```python
from build123d import *

# Parameters (mm, degrees)
SKETCH7_W                       = 41.275
SKETCH7_H                       = 28.575
BOSS_EXTRUDE2_DEPTH             = 50.8
SKETCH31_R                      = 9.525
CUT_EXTRUDE1_DEPTH              = 6.35
FILLET3_R                       = 0.127
F_8_32_TAPPED_HOLE1_D           = 3.4544
F_8_32_TAPPED_HOLE1_DEPTH       = 10.16
F_8_32_TAPPED_HOLE1_TIP         = 1.037806461
F_17_0_173_DIAMETER_HOLE1_D     = 4.3942
F_46_0_081_DIAMETER_HOLE1_D     = 2.0574
F_46_0_081_DIAMETER_HOLE1_DEPTH = 19.066894681
F_46_0_081_DIAMETER_HOLE1_TIP   = 0.618105319


with BuildPart() as part:
    # Sketch7 → Boss-Extrude2 (new body)
    with BuildSketch(Plane(origin=(0, 0, 0), x_dir=(1, 0, 0), z_dir=(0, 1, 0))):
        with Locations((-1.5875, -7.9375)):
            Rectangle(SKETCH7_W, SKETCH7_H)
    extrude(amount=BOSS_EXTRUDE2_DEPTH)

    # Sketch31 → Cut-Extrude1 (cut)
    with BuildSketch(Plane(origin=(0, 0, -6.35), x_dir=(-1, 0, 0), z_dir=(0, 0, -1))):
        with Locations((1.5875, 25.4)):
            Circle(SKETCH31_R)
    extrude(amount=-CUT_EXTRUDE1_DEPTH, mode=Mode.SUBTRACT)

    # Sketch24 → Port Manifold (revolve, cut)
    with BuildSketch(Plane.ZY.offset(1.5875)):
        with BuildLine():
            Line((22.225, 25.4), (22.225, 33.1978))
            Line((22.225, 33.1978), (15.0368, 33.1978))
            Line((15.0368, 33.1978), (14.04146205, 32.9311))
            Line((14.04146205, 32.9311), (8.2804, 32.9311))
            ThreePointArc((8.2804, 32.9311), (8.136715902, 32.871584098), (8.0772, 32.7279))
            Line((8.0772, 32.7279), (8.0772, 29.2735))
            Line((8.0772, 29.2735), (7.637259095, 29.0195))
            Line((7.637259095, 29.0195), (4.7752, 29.0195))
            ThreePointArc((4.7752, 29.0195), (4.631515902, 28.959984098), (4.572, 28.8163))
            Line((4.572, 28.8163), (4.572, 26.034032808))
            Line((4.572, 26.034032808), (3.111576387, 26.04897))
            Line((3.111576387, 26.04897), (-0.714966433, 28.258225527))
            Line((-0.714966433, 28.258225527), (-0.714966433, 25.4))
            Line((-0.714966433, 25.4), (22.225, 25.4))
        make_face()
    revolve(axis=Axis((-1.5875, 25.4, -0.714966433), (0, 0, 1)), mode=Mode.SUBTRACT)

    # Fillet3
    fillet3_edges = [part.edges().sort_by_distance(p)[0] for p in [
        (-1.5875, 24.765967192, 4.572),
    ]]
    fillet(fillet3_edges, radius=FILLET3_R)

    # #8-32 Tapped Hole1
    with Locations(Plane.XY.offset(22.225)):
        with Locations((9.7155, 25.4)):
            Hole(F_8_32_TAPPED_HOLE1_D / 2, depth=F_8_32_TAPPED_HOLE1_DEPTH)
            with Locations((0, 0, -(F_8_32_TAPPED_HOLE1_DEPTH + F_8_32_TAPPED_HOLE1_TIP / 2))):  # 118° drill point
                Cone(0, F_8_32_TAPPED_HOLE1_D / 2, F_8_32_TAPPED_HOLE1_TIP, mode=Mode.SUBTRACT)

    # Sketch29 → 1/8 NPT Tapped Hole1 (revolve, cut)
    with BuildSketch(Plane(origin=(-1.5875, 0, 7.9375), x_dir=(0, 0, -1), z_dir=(1, 0, 0))):
        Polygon((0, 0), (0, 14.217468714), (4.2164, 11.684), (4.2164, 6.858), (4.537401096, 6.858), (4.7427388, 0), align=None)
    revolve(axis=Axis((-1.5875, -6.35, 7.9375), (0, 1, 0)), mode=Mode.SUBTRACT)

    # #17 (0.173) Diameter Hole1 (through all)
    with Locations(Plane.ZY.offset(22.225)):
        with Locations((6.35, 44.45), (15.875, 44.45)):
            Hole(F_17_0_173_DIAMETER_HOLE1_D / 2)

    # #46 (0.081) Diameter Hole1
    with Locations(Plane(origin=(0, 0, 0), x_dir=(-1, 0, 0), z_dir=(0, -1, 0))):
        with Locations((1.5875, -7.9375)):
            Hole(F_46_0_081_DIAMETER_HOLE1_D / 2, depth=F_46_0_081_DIAMETER_HOLE1_DEPTH)
            with Locations((0, 0, -(F_46_0_081_DIAMETER_HOLE1_DEPTH + F_46_0_081_DIAMETER_HOLE1_TIP / 2))):  # 118° drill point
                Cone(0, F_46_0_081_DIAMETER_HOLE1_D / 2, F_46_0_081_DIAMETER_HOLE1_TIP, mode=Mode.SUBTRACT)


solid = part.part
```
Check sheet for the modelled part. Datum: model origin and axes. Units: mm. A direction names the side the tool comes from. Round coordinates to 2 decimals unless told otherwise and drop trailing zeros. Loops run counter-clockwise (first coordinate to the right, second up) from the corner with the lowest first, then second, coordinate; pieces in that order, holes last. Notation, with made-up numbers: (16, 71) - (26, 71) arc R8 cw to (26, 82) - close; hole circle Ø3 at (-24, 25.5). An arc over 180 degrees is marked (long way). Write item = value, one per line. Start each with the question number.
Q1. Access from +Z, -Z, +X, -X, +Y, -Y to the whole of each face (thin tool, end or side, straight path). Record for faces 1 (the face through (-4, 23, 0)), 2 (the face through (-1.721, 16.371, 6.918)), 3 (the face through (2, 29, 8.077)).
Q2. Section check B-B (x = -14.5). Record the boundary of the cut face in (y, z) (3 decimals).
Q3. Section check D-D (z = 18.75). Count the separate pieces of the cut face and the enclosed holes in it, plus the area to 3 significant figures.
Q4. Section check A-A (y = 44.45). Record the boundary of the cut face in (x, z) (3 decimals).
Q5. Depth check by flat-ended pin: P1, Ø1.6, axis at x = -1.59, z = 7.94, coming from the -Y side; P2, Ø6.5, axis at x = -1.59, y = 25.4, coming from the +Z side; P3, Ø15, axis at x = -2, y = 23.5, coming from the -Z side. Enter the tip coordinate at first touch or a pass-through.
Q6. Thickness scan on L1, parallel to X at y = 5.5, z = 9.75 (3 decimals); L2, parallel to X at y = 25.5, z = 17.5 (3 decimals); L3, parallel to X at y = 25.5, z = -3.5 (3 decimals). Record the ranges inside material, lowest first.
Q7. Release check for a two-part mould opening along Y. For faces 4 (the face through (-1.299, 46.628, 6.636)), 5 (the face through (0.027, 9.237, 4.043)), 6 (the face through (-2.98, 3.38, 3.51)) record: pulls with the +Y half, pulls with the -Y half, needs draft (parallel to the pull), parting line crosses it, or undercut.
Derived:
q1.face_1 = -Z
q1.face_2 = -Y
q1.face_3 = +Z
q2.outline = (0, -6.35) - (50.8, -6.35) - (50.8, 22.225) - (0, 22.225) - close; hole circle Ø4.394 at (44.45, 6.35); hole circle Ø4.394 at (44.45, 15.875)
q3.separate_pieces = 1
q3.enclosed_holes = 2
q3.area = 1,900 mm^2
q4.outline = (-22.225, -6.35) - (19.05, -6.35) - (19.05, 4.153) - (-22.225, 4.153) - close; (-22.225, 8.547) - (19.05, 8.547) - (19.05, 13.678) - (-22.225, 13.678) - close; (-22.225, 18.072) - (19.05, 18.072) - (19.05, 22.225) - (-22.225, 22.225) - close
q5.P1 = 19.2
q5.P2 = 4.57
q5.P3 = 0
q6.L1 = -22.225 to -5.791, 2.616 to 19.05
q6.L2 = -22.225 to -9.385, 6.21 to 7.991, 11.44 to 19.05
q6.L3 = -22.225 to -11.112, 7.937 to 19.05
q7.face_4 = undercut
q7.face_5 = needs draft
q7.face_6 = pulls with the -Y half
